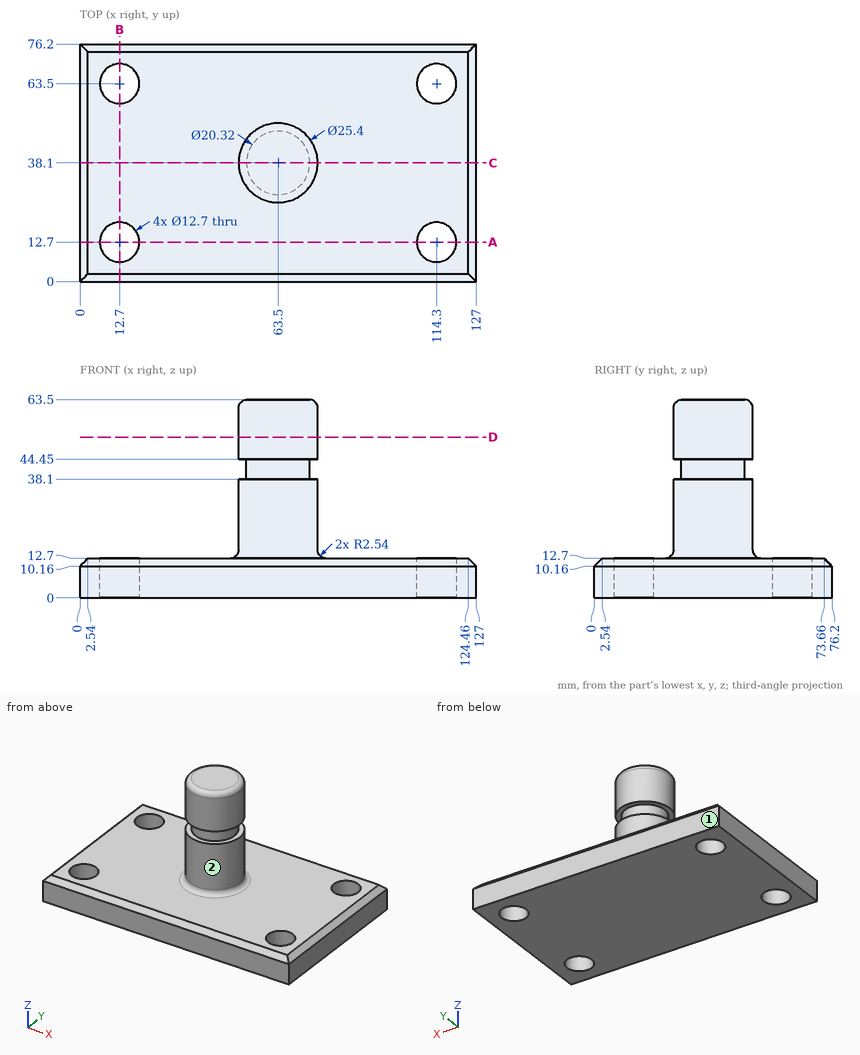
Study the drawing (mm; zero at the part's minimum x, y, z) and answer. A direction names the side the tool comes from. Give positions to 0.01 mm unless a question says otherwise; leave off trailing zeros. Write each loop counter-clockwise with the first axis right and the second up, starting at its lowest first coordinate (ties: lowest second). Pieces come first, ordered by that corner, then holes.
(1) The part is cut by section C-C on y = 38.1. Write down the section's boundary in (x, z), plus the area to 3 significant figures.
Final values:
outline: (0, 0) - (127, 0) - (127, 10.16) - (124.46, 12.7) - (78.74, 12.7) arc R2.54 cw to (76.2, 15.24) - (76.2, 38.1) - (73.66, 38.1) - (73.66, 44.45) - (76.2, 44.45) - (76.2, 60.96) arc R2.54 ccw to (73.66, 63.5) - (53.34, 63.5) arc R2.54 ccw to (50.8, 60.96) - (50.8, 44.45) - (53.34, 44.45) - (53.34, 38.1) - (50.8, 38.1) - (50.8, 15.24) arc R2.54 cw to (48.26, 12.7) - (2.54, 12.7) - (0, 10.16) - close
area: 2,860 mm2
(2) The part is cut by section D-D on z = 51.5. Write down the section's boundary in (x, y), plus the area to 3 significant figures.
Final values:
outline: circle Ø25.4 at (63.5, 38.1)
area: 507 mm2
(3) Flat-ended cylindrical pins translate along their axes: pin 1 Ø1.5 at (x, z) = (73.5, 14.5) entering from +Y; pin 2 Ø11.5 at (x, y) = (114.3, 12.7) entering from +Z; pin 3 Ø2 at (y, z) = (28.5, 46.5) entering from -X; pin 4 Ø20.5 at (x, y) = (12.7, 12.7) entering from +Z. Find the tip coordinate at first contact, or state that the pin passes through.
Final values:
pin 1: stops at y = 47.07
pin 2: passes through
pin 3: stops at x = 54.15
pin 4: stops at z = 12.7
(4) The part is cut by section A-A on y = 12.7. Write down the section's boundary in (x, z).
Final values:
outline: (0, 0) - (6.35, 0) - (6.35, 12.7) - (2.54, 12.7) - (0, 10.16) - close; (19.05, 0) - (107.95, 0) - (107.95, 12.7) - (19.05, 12.7) - close; (120.65, 0) - (127, 0) - (127, 10.16) - (124.46, 12.7) - (120.65, 12.7) - close
(5) Which of the six approach directions +Z, -Z, +X, -X, +Y, -Y give full straight-line access (tool end or side, diameter ignored) to the marked faces 1 and 2?
Final values:
face 1: +Z, -Z, +X, -X, +Y
face 2: +Z
(6) Straight lines are drawn through the part: line 1 (Y direction, x = 12.7, z = 3); line 2 (X direction, y = 12, z = 9); line 3 (Z direction, x = 18, y = 28). For each, find the intervals that lie inside material, in ascending order.
Final values:
line 1: y = 0 to 6.35, 19.05 to 57.15, 69.85 to 76.2
line 2: x = 0 to 6.39, 19.01 to 107.99, 120.61 to 127
line 3: z = 0 to 12.7
(7) The part is cut by section B-B on x = 12.7. Write down the section's boundary in (y, z).
Final values:
outline: (0, 0) - (6.35, 0) - (6.35, 12.7) - (2.54, 12.7) - (0, 10.16) - close; (19.05, 0) - (57.15, 0) - (57.15, 12.7) - (19.05, 12.7) - close; (69.85, 0) - (76.2, 0) - (76.2, 10.16) - (73.66, 12.7) - (69.85, 12.7) - close
